```python
from build123d import *
from build123d.topology import SkipClean

# Parameters (mm, degrees)
SKETCH2_R                = 81.32791599
SKETCH2_R_2              = 20
BOSS_EXTRUDE1_DEPTH      = 3
BOSS_EXTRUDE1_DEPTH_BACK = 63
SKETCH3_R                = 70
CUT_EXTRUDE1_DEPTH       = 30
SKETCH4_R                = 70
CUT_EXTRUDE2_DEPTH       = 20
CUT_EXTRUDE3_DEPTH       = 20
CUT_EXTRUDE3_DEPTH_BACK  = 30
SKETCH6_R                = 2.5934664
BOSS_EXTRUDE2_DEPTH      = 2


with BuildPart() as part:
    # Sketch1 → Revolve1 (revolve)
    with BuildSketch(Plane.XY, mode=Mode.PRIVATE) as revolve1_sk:
        Polygon((25, 100), (25, 75), (30, 75), (30, 105), (29, 105), (29, 105.702764037), (26, 105.702764037), (26, 105), (22, 105), (22, 105.702764037), (19, 105.702764037), (19, 105), (15, 105), (15, 105.702764037), (12, 105.702764037), (12, 105), (8, 105), (8, 105.702764037), (5, 105.702764037), (5, 105), (1, 105), (1, 105.702764037), (-2, 105.702764037), (-2, 105), (-6, 105), (-6, 105.702764037), (-9, 105.702764037), (-9, 105), (-13, 105), (-13, 105.702764037), (-16, 105.702764037), (-16, 105), (-20, 105), (-20, 105.702764037), (-23, 105.702764037), (-23, 105), (-27, 105), (-27, 105.702764037), (-30, 105.702764037), (-30, 75), (-25, 75), (-25, 100), align=None)
    revolve(revolve1_sk.sketch.rotate(Axis((-60.37659433, 0, 0), (1, 0, 0)), 90), axis=Axis((-60.37659433, 0, 0), (1, 0, 0)))

    # Sketch2 → Boss-Extrude1 (add, two sides)
    with BuildSketch(Plane(origin=(30, 0, 0), x_dir=(0, 0, -1), z_dir=(1, 0, 0))) as boss_extrude1_sk:
        Circle(SKETCH2_R)
        Circle(SKETCH2_R_2, mode=Mode.SUBTRACT)
    extrude(amount=BOSS_EXTRUDE1_DEPTH)
    extrude(boss_extrude1_sk.sketch, amount=-BOSS_EXTRUDE1_DEPTH_BACK)

    # Sketch3 → Cut-Extrude1 (cut)
    with BuildSketch(Plane(origin=(33, 0, 0), x_dir=(0, 0, -1), z_dir=(1, 0, 0))):
        Circle(SKETCH3_R)
    extrude(amount=-CUT_EXTRUDE1_DEPTH, mode=Mode.SUBTRACT)

    # Sketch4 → Cut-Extrude2 (cut)
    with BuildSketch(Plane.ZY.offset(33)):
        with Locations(Location((0, 0, 0), (0, 0, 180))):
            Circle(SKETCH4_R)
    extrude(amount=-CUT_EXTRUDE2_DEPTH, mode=Mode.SUBTRACT)

    # Sketch5 → Cut-Extrude3 (cut, two sides)
    with SkipClean():  # the faces are left unmerged after this step: merging them gives an invalid solid
        with BuildSketch(Plane(origin=(3, 0, 0), x_dir=(0, 0, -1), z_dir=(1, 0, 0))) as cut_extrude3_sk:
            with BuildLine():
                ThreePointArc((-57.241605299, 40.291421206), (-47.954627948, 0), (-57.241605299, -40.291421206))
                ThreePointArc((-57.241605299, -40.291421206), (-70, 0), (-57.241605299, 40.291421206))
            make_face()
            with BuildLine():
                ThreePointArc((-43.034620977, -55.208888753), (0, -44.913138925), (43.034620977, -55.208888753))
                ThreePointArc((43.034620977, -55.208888753), (0, -70), (-43.034620977, -55.208888753))
            make_face()
            with BuildLine():
                ThreePointArc((57.241605299, 40.291421206), (47.954627948, 0), (57.241605299, -40.291421206))
                ThreePointArc((57.241605299, -40.291421206), (70, 0), (57.241605299, 40.291421206))
            make_face()
            with BuildLine():
                ThreePointArc((-43.034620977, 55.208888753), (0, 44.913138925), (43.034620977, 55.208888753))
                ThreePointArc((43.034620977, 55.208888753), (0, 70), (-43.034620977, 55.208888753))
            make_face()
        extrude(amount=CUT_EXTRUDE3_DEPTH, mode=Mode.SUBTRACT)
        extrude(cut_extrude3_sk.sketch, amount=-CUT_EXTRUDE3_DEPTH_BACK, mode=Mode.SUBTRACT)

    # Sketch6 → Boss-Extrude2 (add)
    with BuildSketch(Plane.ZY.offset(13)):
        with Locations((-33.454711328, 29.112032454)):
            Circle(SKETCH6_R)
    extrude(amount=BOSS_EXTRUDE2_DEPTH)


solid = part.part
```
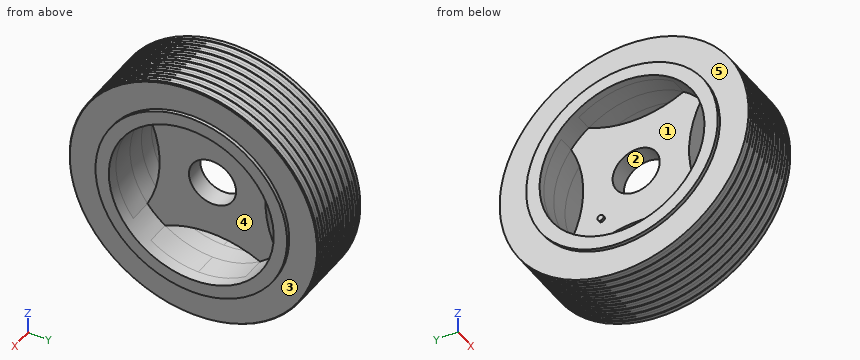
Can you work these out from the model? Positions are in its coordinate system, mm. Face numbers are marked on the shaded views. A direction names the side the tool comes from. Give positions to 0.01 mm unless a question says otherwise; leave off trailing zeros. Use a Markdown table: item, result. Add a question column.
Q1. On a 3-axis mill with a long thin cutter (end or side, diameter ignored), from which of +Z, -Z, +X, -X, +Y, -Y can I reach the whole of each face in a straight line? I mean the marked faces 4 and 5. Say none if no direction works.
Q2. Please list where these lines run through material, in increasing order: line 1 along Y through (x, z) = (-10, 0); line 2 along X through (y, z) = (-78, -34); line 3 along Y through (x, z) = (20, -55).
Q3. If we section it at A-A on z = 0: Count the separate pieces of the cut face and the enclosed holes in it, plus the area to 3 significant figures.
Q4. If we mould it in two halves opening along Z, with no side actions, what happens to the marked faces 1, 2 and 3? For each: released by +Z, released by -Z, zero draft, split by the parting line, or undercut.
Q5. I'm going to push flat-ended pins straight in: pin 1 (10 mm diameter, centred on x = -9, z = 58, fed in from -Y); pin 2 (12 mm diameter, centred on x = -14, y = -27.5, fed in from -Z); pin 3 (4 mm diameter, centred on y = 29.5, z = -33.5, fed in from -X). Where does each tip first touch, or does it pass through?
Answers follow:
| question | item | result |
|---|---|---|
| 1 | face 4 | +X |
| 1 | face 5 | -X |
| 2 | line 1 | y = -105 to -100, -81.33 to -70, -44.91 to -20, 20 to 44.91, 70 to 81.33, 100 to 105 |
| 2 | line 2 | x = -30 to -25, 25 to 30 |
| 2 | line 3 | y = -90.27 to -83.52, -59.91 to -43.3, 43.3 to 59.91, 83.52 to 90.27 |
| 3 | separate pieces | 4 |
| 3 | enclosed holes | 2 |
| 3 | area | 3,300 mm^2 |
| 4 | face 1 | undercut |
| 4 | face 2 | undercut |
| 4 | face 3 | zero draft |
| 5 | pin 1 | stops at y = -91.46 |
| 5 | pin 2 | stops at z = -103.49 |
| 5 | pin 3 | stops at x = -15 |
